Could you check a few things on this model? Use its own coordinates, in mm. A direction names the side the tool comes from. Give positions to 0.01 mm unless a question says otherwise; leave off trailing zeros. Order: outer loops, then holes, each group sorted by start corner. A loop starts at its lowest first (then second) coordinate and runs counter-clockwise, first axis right, second up.
from build123d import *

# Parameters (mm, degrees)
F1_DEPTH = 6.35
F2_DEPTH = 25.4
F3_R     = 3.175
F4_DEPTH = 17.78


with BuildPart() as f1:
    # F0 (on Right) → F1 (new body)
    with BuildSketch(Plane.YZ):
        with BuildLine():
            ThreePointArc((1.85e-08, -15.875), (-13.1884011008, -8.836385087), (-14.6819263939, 6.0379352732))
            ThreePointArc((-14.6819263939, 6.0379352732), (-18.8258986856, 4.3091372138), (-20.5546969332, 8.4531094269))
            ThreePointArc((-20.5546969332, 8.4531094269), (-18.4637615858, -12.370939055), (-8.66e-08, -22.225))
            ThreePointArc((-8.66e-08, -22.225), (-3.175, -19.0499999474), (1.85e-08, -15.875))
        make_face()
        with BuildLine():
            ThreePointArc((20.7933116087, 7.2455224835), (18.2337795642, 4.1307473398), (14.6819262886, 6.0379355294))
            ThreePointArc((14.6819262886, 6.0379355294), (15.5738756389, 3.0773401802), (15.875, 0))
            ThreePointArc((15.875, 0), (11.2253201579, -11.2253201448), (1.85e-08, -15.875))
            ThreePointArc((1.85e-08, -15.875), (2.2450640368, -16.8049359763), (3.175, -19.05))
            ThreePointArc((3.175, -19.05), (2.2450639997, -21.2950640609), (-8.66e-08, -22.225))
            ThreePointArc((-8.66e-08, -22.225), (15.7154481813, -15.7154482425), (22.225, 0))
            ThreePointArc((22.225, 0), (21.803425923, 4.3082761076), (20.5546969161, 8.4531094685))
            ThreePointArc((20.5546969161, 8.4531094685), (20.7330867492, 7.8609904554), (20.7933116087, 7.2455224835))
        make_face()
        with BuildLine():
            Line((2.54, 15.6704826027), (2.54, 12.4434078933))
            ThreePointArc((2.54, 12.4434078933), (5.9587621309, 11.2153089065), (8.89, 9.0696141042))
            Line((8.89, 9.0696141042), (8.89, 13.1523201375))
            ThreePointArc((8.89, 13.1523201375), (5.8520518239, 14.7570022176), (2.54, 15.6704826027))
        make_face()
        with BuildLine():
            Line((2.54, 25.2726809025), (2.54, 23.7934423739))
            Line((2.54, 23.7934423739), (8.89, 23.7934423739))
            ThreePointArc((8.89, 23.7934423739), (5.7626609874, 24.7376583036), (2.54, 25.2726809025))
        make_face()
        with BuildLine():
            Line((-8.89, 23.7934423739), (-2.54, 23.7934423739))
            Line((-2.54, 23.7934423739), (-2.54, 25.2726809025))
            ThreePointArc((-2.54, 25.2726809025), (-5.7626609874, 24.7376583036), (-8.89, 23.7934423739))
        make_face()
        with BuildLine():
            ThreePointArc((-8.89, 9.0696141042), (-5.9587621309, 11.2153089065), (-2.54, 12.4434078933))
            Line((-2.54, 12.4434078933), (-2.54, 15.6704826027))
            ThreePointArc((-2.54, 15.6704826027), (-5.8520518239, 14.7570022176), (-8.89, 13.1523201375))
            Line((-8.89, 13.1523201375), (-8.89, 9.0696141042))
        make_face()
        with BuildLine():
            Line((-8.89, 0), (-6.35, 0))
            ThreePointArc((-6.35, 0), (-5.3127911685, 3.4780382402), (-2.54, 5.8198711326))
            Line((-2.54, 5.8198711326), (-2.54, 12.4434078933))
            ThreePointArc((-2.54, 12.4434078933), (-5.9587621309, 11.2153089065), (-8.89, 9.0696141042))
            Line((-8.89, 9.0696141042), (-8.89, 0))
        make_face()
        with BuildLine():
            Line((8.89, 0), (6.35, 0))
            ThreePointArc((6.35, 0), (0, -6.35), (-6.35, 0))
            Line((-6.35, 0), (-8.89, 0))
            Line((-8.89, 0), (-8.89, 9.0696141042))
            ThreePointArc((-8.89, 9.0696141042), (-4.9186888497, -11.7088214608), (12.7, 0))
            ThreePointArc((12.7, 0), (11.7088214608, 4.9186888497), (8.89, 9.0696141042))
            Line((8.89, 9.0696141042), (8.89, 0))
        make_face()
        with BuildLine():
            ThreePointArc((2.54, 5.8198711326), (5.3127911685, 3.4780382402), (6.35, 0))
            Line((6.35, 0), (8.89, 0))
            Line((8.89, 0), (8.89, 9.0696141042))
            ThreePointArc((8.89, 9.0696141042), (5.9587621309, 11.2153089065), (2.54, 12.4434078933))
            Line((2.54, 12.4434078933), (2.54, 5.8198711326))
        make_face()
        with BuildLine():
            ThreePointArc((-13.7481533134, 7.937499951), (-11.6155104819, 10.8210693208), (-8.89, 13.1523201375))
            Line((-8.89, 13.1523201375), (-8.89, 20.3695489641))
            ThreePointArc((-8.89, 20.3695489641), (-14.8105289031, 16.5710246699), (-19.247414709, 11.1124998097))
            ThreePointArc((-19.247414709, 11.1124998097), (-15.67603358, 12.5918145269), (-13.3227839421, 9.525))
            ThreePointArc((-13.3227839421, 9.525), (-13.4309694509, 8.7032495045), (-13.7481533134, 7.937499951))
        make_face()
        with BuildLine():
            Line((8.89, 13.1523201375), (8.89, 9.0696141042))
            ThreePointArc((8.89, 9.0696141042), (11.7088214608, 4.9186888497), (12.7, 0))
            ThreePointArc((12.7, 0), (-4.9186888497, -11.7088214608), (-8.89, 9.0696141042))
            Line((-8.89, 9.0696141042), (-8.89, 13.1523201375))
            ThreePointArc((-8.89, 13.1523201375), (-11.6155104819, 10.8210693208), (-13.7481533134, 7.937499951))
            ThreePointArc((-13.7481533134, 7.937499951), (-14.2467345217, 7.003297828), (-14.6819263939, 6.0379352732))
            ThreePointArc((-14.6819263939, 6.0379352732), (-13.1884011008, -8.836385087), (1.85e-08, -15.875))
            ThreePointArc((1.85e-08, -15.875), (11.2253201579, -11.2253201448), (15.875, 0))
            ThreePointArc((15.875, 0), (15.5738756389, 3.0773401802), (14.6819262886, 6.0379355294))
            ThreePointArc((14.6819262886, 6.0379355294), (14.2467344349, 7.0032980045), (13.7481532552, 7.9375000518))
            ThreePointArc((13.7481532552, 7.9375000518), (11.6155104422, 10.8210693634), (8.89, 13.1523201375))
        make_face()
        with BuildLine():
            Line((8.89, 23.7934423739), (8.89, 20.3695489641))
            ThreePointArc((8.89, 20.3695489641), (14.8105289204, 16.5710246545), (19.2474147322, 11.1124997695))
            ThreePointArc((19.2474147322, 11.1124997695), (19.9454283511, 9.804616917), (20.5546969161, 8.4531094685))
            ThreePointArc((20.5546969161, 8.4531094685), (21.803425923, 4.3082761076), (22.225, 0))
            ThreePointArc((22.225, 0), (15.7154481813, -15.7154482425), (-8.66e-08, -22.225))
            ThreePointArc((-8.66e-08, -22.225), (-18.4637615858, -12.370939055), (-20.5546969332, 8.4531094269))
            ThreePointArc((-20.5546969332, 8.4531094269), (-19.9454283508, 9.8046169177), (-19.247414709, 11.1124998097))
            ThreePointArc((-19.247414709, 11.1124998097), (-14.8105289031, 16.5710246699), (-8.89, 20.3695489641))
            Line((-8.89, 20.3695489641), (-8.89, 23.7934423739))
            ThreePointArc((-8.89, 23.7934423739), (-14.4802278988, -20.8682294409), (25.4, 0))
            ThreePointArc((25.4, 0), (20.8682294409, 14.4802278988), (8.89, 23.7934423739))
        make_face()
        with BuildLine():
            ThreePointArc((-8.89, 20.3695489641), (-5.7785902794, 21.4606271899), (-2.54, 22.0793800864))
            Line((-2.54, 22.0793800864), (-2.54, 23.7934423739))
            Line((-2.54, 23.7934423739), (-8.89, 23.7934423739))
            Line((-8.89, 23.7934423739), (-8.89, 20.3695489641))
        make_face()
        with BuildLine():
            ThreePointArc((-8.89, 13.1523201375), (-5.8520518239, 14.7570022176), (-2.54, 15.6704826027))
            Line((-2.54, 15.6704826027), (-2.54, 22.0793800864))
            ThreePointArc((-2.54, 22.0793800864), (-5.7785902794, 21.4606271899), (-8.89, 20.3695489641))
            Line((-8.89, 20.3695489641), (-8.89, 13.1523201375))
        make_face()
        with BuildLine():
            Line((2.54, 22.0793800864), (2.54, 15.6704826027))
            ThreePointArc((2.54, 15.6704826027), (5.8520518239, 14.7570022176), (8.89, 13.1523201375))
            Line((8.89, 13.1523201375), (8.89, 20.3695489641))
            ThreePointArc((8.89, 20.3695489641), (5.7785902794, 21.4606271899), (2.54, 22.0793800864))
        make_face()
        with BuildLine():
            Line((2.54, 23.7934423739), (2.54, 22.0793800864))
            ThreePointArc((2.54, 22.0793800864), (5.7785902794, 21.4606271899), (8.89, 20.3695489641))
            Line((8.89, 20.3695489641), (8.89, 23.7934423739))
            Line((8.89, 23.7934423739), (2.54, 23.7934423739))
        make_face()
        with BuildLine():
            Line((8.89, 20.3695489641), (8.89, 13.1523201375))
            ThreePointArc((8.89, 13.1523201375), (11.6155104422, 10.8210693634), (13.7481532552, 7.9375000518))
            ThreePointArc((13.7481532552, 7.9375000518), (14.9102840832, 12.2746307385), (19.2474147322, 11.1124997695))
            ThreePointArc((19.2474147322, 11.1124997695), (14.8105289204, 16.5710246545), (8.89, 20.3695489641))
        make_face()
    extrude(amount=F1_DEPTH)

    # F0 (on Right) → F2 (join)
    with BuildSketch(Plane.YZ):
        with BuildLine():
            ThreePointArc((2.54, 5.8198711326), (5.3127911685, 3.4780382402), (6.35, 0))
            Line((6.35, 0), (8.89, 0))
            Line((8.89, 0), (8.89, 9.0696141042))
            ThreePointArc((8.89, 9.0696141042), (5.9587621309, 11.2153089065), (2.54, 12.4434078933))
            Line((2.54, 12.4434078933), (2.54, 5.8198711326))
        make_face()
        with BuildLine():
            Line((2.54, 15.6704826027), (2.54, 12.4434078933))
            ThreePointArc((2.54, 12.4434078933), (5.9587621309, 11.2153089065), (8.89, 9.0696141042))
            Line((8.89, 9.0696141042), (8.89, 13.1523201375))
            ThreePointArc((8.89, 13.1523201375), (5.8520518239, 14.7570022176), (2.54, 15.6704826027))
        make_face()
        with BuildLine():
            ThreePointArc((-8.89, 9.0696141042), (-5.9587621309, 11.2153089065), (-2.54, 12.4434078933))
            Line((-2.54, 12.4434078933), (-2.54, 15.6704826027))
            ThreePointArc((-2.54, 15.6704826027), (-5.8520518239, 14.7570022176), (-8.89, 13.1523201375))
            Line((-8.89, 13.1523201375), (-8.89, 9.0696141042))
        make_face()
        with BuildLine():
            Line((-8.89, 0), (-6.35, 0))
            ThreePointArc((-6.35, 0), (-5.3127911685, 3.4780382402), (-2.54, 5.8198711326))
            Line((-2.54, 5.8198711326), (-2.54, 12.4434078933))
            ThreePointArc((-2.54, 12.4434078933), (-5.9587621309, 11.2153089065), (-8.89, 9.0696141042))
            Line((-8.89, 9.0696141042), (-8.89, 0))
        make_face()
        with BuildLine():
            Line((8.89, 0), (6.35, 0))
            ThreePointArc((6.35, 0), (0, -6.35), (-6.35, 0))
            Line((-6.35, 0), (-8.89, 0))
            Line((-8.89, 0), (-8.89, 9.0696141042))
            ThreePointArc((-8.89, 9.0696141042), (-4.9186888497, -11.7088214608), (12.7, 0))
            ThreePointArc((12.7, 0), (11.7088214608, 4.9186888497), (8.89, 9.0696141042))
            Line((8.89, 9.0696141042), (8.89, 0))
        make_face()
        with BuildLine():
            Line((-8.89, 23.7934423739), (-2.54, 23.7934423739))
            Line((-2.54, 23.7934423739), (-2.54, 25.2726809025))
            ThreePointArc((-2.54, 25.2726809025), (-5.7626609874, 24.7376583036), (-8.89, 23.7934423739))
        make_face()
        with BuildLine():
            Line((2.54, 25.2726809025), (2.54, 23.7934423739))
            Line((2.54, 23.7934423739), (8.89, 23.7934423739))
            ThreePointArc((8.89, 23.7934423739), (5.7626609874, 24.7376583036), (2.54, 25.2726809025))
        make_face()
        with BuildLine():
            ThreePointArc((-8.89, 13.1523201375), (-5.8520518239, 14.7570022176), (-2.54, 15.6704826027))
            Line((-2.54, 15.6704826027), (-2.54, 22.0793800864))
            ThreePointArc((-2.54, 22.0793800864), (-5.7785902794, 21.4606271899), (-8.89, 20.3695489641))
            Line((-8.89, 20.3695489641), (-8.89, 13.1523201375))
        make_face()
        with BuildLine():
            ThreePointArc((-8.89, 20.3695489641), (-5.7785902794, 21.4606271899), (-2.54, 22.0793800864))
            Line((-2.54, 22.0793800864), (-2.54, 23.7934423739))
            Line((-2.54, 23.7934423739), (-8.89, 23.7934423739))
            Line((-8.89, 23.7934423739), (-8.89, 20.3695489641))
        make_face()
        with BuildLine():
            Line((2.54, 22.0793800864), (2.54, 15.6704826027))
            ThreePointArc((2.54, 15.6704826027), (5.8520518239, 14.7570022176), (8.89, 13.1523201375))
            Line((8.89, 13.1523201375), (8.89, 20.3695489641))
            ThreePointArc((8.89, 20.3695489641), (5.7785902794, 21.4606271899), (2.54, 22.0793800864))
        make_face()
        with BuildLine():
            Line((2.54, 23.7934423739), (2.54, 22.0793800864))
            ThreePointArc((2.54, 22.0793800864), (5.7785902794, 21.4606271899), (8.89, 20.3695489641))
            Line((8.89, 20.3695489641), (8.89, 23.7934423739))
            Line((8.89, 23.7934423739), (2.54, 23.7934423739))
        make_face()
    extrude(amount=F2_DEPTH)

    # F3 (on face) → F4 (cut, through all)
    with BuildSketch(Plane(origin=(0, 8.89, 0), x_dir=(-1, 0, 0), z_dir=(0, 1, 0))):
        with Locations((-15.875, 16.4315282391)):
            Circle(F3_R)
    extrude(amount=-F4_DEPTH, mode=Mode.SUBTRACT)


solid = f1.part
Item 1: Please list where these lines run through material, in increasing order: line 1 along Y through (x, z) = (12.75, 0); line 2 along Y through (x, z) = (2, 11); line 3 along Z through (x, y) = (15.5, 5).
Findings:
line 1: y = -12.7 to -6.35, 6.35 to 12.7
line 2: y = -22.89 to -19.31, -13.69 to -2.54, 2.54 to 13.69, 19.31 to 22.89
line 3: z = -11.67 to -3.91, 3.91 to 13.28, 19.58 to 24.9
Item 2: For faces 1 (the flat face through (12.5, 2.54, 15.7)), 2 (the cylindrical face through (3.131, -19.955, 9.786)), 3 (the flat face through (16, 8.89, 13)), which set-ups out of +Z, -Z, +X, -X, +Y, -Y let a thin tool reach every point of the face, with its end or its side?
Findings:
face 1: +Z, +X, -X
face 2: +X, -X
face 3: +Z, +X, +Y
Item 3: We'd pull the mould along Y, two halves only. Please class faces 4 (the cylindrical face through (3.13, -14.24, 7.02)), 5 (the cylindrical face through (3.13, 14.85, 12.24)), 6 (the flat face through (16, -8.89, 20)), 7 (the flat face through (6.35, -6, -11.4)): +Y half, -Y half, draft (parallel to the pull), parting line (faces both ways), or undercut.
Findings:
face 4: undercut
face 5: undercut
face 6: -Y half
face 7: draft
Item 4: Imagine slicing it at B-B on z = -12. List the corners of the cut face in (x, y) for me.
Findings:
outline: (0, -22.39) - (6.35, -22.39) - (6.35, -4.16) - (25.4, -4.16) - (25.4, 4.16) - (6.35, 4.16) - (6.35, 22.39) - (0, 22.39) - close
Item 5: Imagine slicing it at A-A on y = 10. List the corners of the cut face in (x, z) for me, then the cut area to 3 significant figures.
Findings:
outline: (0, -23.35) - (6.35, -23.35) - (6.35, -7.83) - (25.4, -7.83) - (25.4, 7.83) - (6.35, 7.83) - (6.35, 23.35) - (0, 23.35) - close
area: 595 mm2
Item 6: For pin 1 (3 mm diameter, centred on y = 1.5, z = -15.5, fed in from +X); pin 2 (1 mm diameter, centred on x = 20.5, z = -7, fed in from +Y); pin 3 (4 mm diameter, centred on x = 9, z = 2.5, fed in from -Y), each with a flat end and sliding along its axis, tell me the tip position at first contact or that it passes through.
Findings:
pin 1: stops at x = 6.35
pin 2: stops at y = 10.91
pin 3: stops at y = -12.69
